Design review of the part built by this model. Coordinates are the model's own, in mm. Face numbers are marked on the shaded views. A direction names the side the tool comes from. Round coordinates to 2 decimals unless told otherwise and drop trailing zeros. Loops run counter-clockwise (first coordinate to the right, second up) from the corner with the lowest first, then second, coordinate; pieces in that order, holes last. Notation, with made-up numbers: (73.5, -13) -> (103.5, -13) arc R18 cw to (103.5, -6) -> close; hole circle Ø7 at (77, 48.25). An arc over 180 degrees is marked (long way). Write each question's results on one line, items separated by ' | '. Start each with the question number.
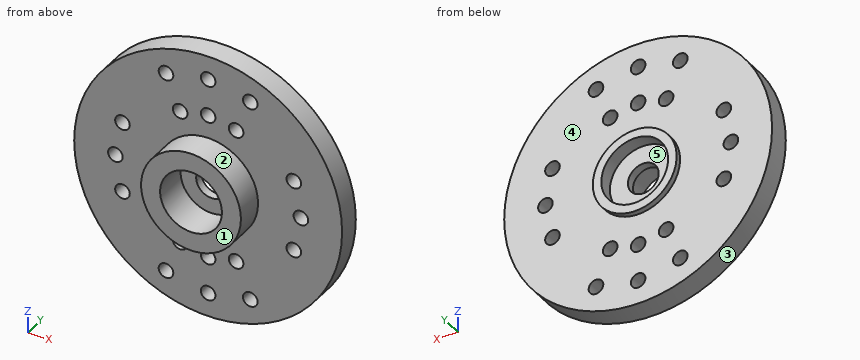
Autodesk Inventor part; units mm, degrees
ref_plane "YZ Plane" through (0, 0, 0) normal (1, 0, 0) x (0, 1, 0)
ref_plane "XZ Plane" through (0, 0, 0) normal (0, 1, 0) x (-1, 0, 0)
ref_plane "XY Plane" through (0, 0, 0) normal (0, 0, 1) x (1, 0, 0)
sketch "Sketch1" plane through (0, 0, 0) normal (0, 1, 0) x (-1, 0, 0)
  circle A0 centre (0, 0) radius 11.915
  dimension "d0" = 23.83
extrude "Extrusion1" add sketch "Sketch1" along normal blind 2
sketch "Sketch2" plane through (0, 2, 0) normal (0, 1, 0) x (1, 0, 0)
  circle A0 centre (0, 6.5) radius 0.65
  line L0 (0, 0) -> (6.5, 0) construction
  circle A1 centre (2.4874, 6.0052) radius 0.65
  circle A2 centre (8.25, 0) radius 0.65
  line L1 (0, 0) -> (8.25, 0) construction
  circle A3 centre (7.622, 3.1571) radius 0.65
  circle A4 centre (0, 9.8) radius 0.65
  line L2 (0, 0) -> (9.8, 0) construction
  circle A5 centre (3.7503, 9.054) radius 0.65
  circle A6 centre (0, 0) radius 11.915
  circle A7 centre (-2.4874, 6.0052) radius 0.65
  circle A8 centre (-8.25, 0) radius 0.65
  circle A9 centre (-7.622, 3.1571) radius 0.65
  circle A10 centre (-3.7503, 9.054) radius 0.65
  circle A11 centre (0, -6.5) radius 0.65
  circle A12 centre (2.4874, -6.0052) radius 0.65
  circle A13 centre (7.622, -3.1571) radius 0.65
  circle A14 centre (0, -9.8) radius 0.65
  circle A15 centre (3.7503, -9.054) radius 0.65
  circle A16 centre (-3.7503, -9.054) radius 0.65
  circle A17 centre (-2.4874, -6.0052) radius 0.65
  circle A18 centre (-7.622, -3.1571) radius 0.65
  dimension "d5" = 1.3
  dimension "d8" = 1.3
  dimension "d10" = 1.3
  dimension "d13" = 1.3
  dimension "d15" = 1.3
  dimension "d18" = 1.3
extrude "Extrusion2" cut sketch "Sketch2" against normal blind 2 contours A0 | A1 | A2 | A3 | A4 | A5 | A7 | A8 | A9 | A10 | A11 | A12 | A13 | A14 | A15 | A16 | A17 | A18
sketch "Sketch3" plane through (0, 2, 0) normal (0, 1, 0) x (1, 0, 0)
  circle A0 centre (0, 0) radius 3.73
  dimension "d21" = 7.46
extrude "Extrusion3" add sketch "Sketch3" along normal blind 0.5
sketch "Sketch4" plane through (0, 2.5, 0) normal (0, 1, 0) x (1, 0, 0)
  circle A0 centre (0, 0) radius 2.97
  dimension "d24" = 5.94
extrude "Extrusion4" cut sketch "Sketch4" against normal blind 1.25
sketch "Sketch5" plane through (0, 1.25, 0) normal (0, 1, 0) x (1, 0, 0)
  circle A0 centre (0, 0) radius 1.37
  dimension "d27" = 2.74
extrude "Extrusion5" cut sketch "Sketch5" against normal blind 0.75
sketch "Sketch6" plane through (0, 0, 0) normal (0, -1, 0) x (1, 0, 0)
  circle A0 centre (0, 0) radius 4.44
  dimension "d30" = 8.88
extrude "Extrusion6" add sketch "Sketch6" along normal blind 2.5
sketch "Sketch7" plane through (0, -2.5, 0) normal (0, -1, 0) x (1, 0, 0)
  circle A0 centre (0, 0) radius 2.75
  dimension "d33" = 5.5
extrude "Extrusion7" cut sketch "Sketch7" against normal blind 3
properties part number "MMAE 232 Assignment 2_White Circle - Dylan Tamras"
1) To check wall thickness, follow line 1 (Z direction, x = 0, y = 1.5) (3 decimals); line 2 (Z direction, x = 0, y = 1.05) (3 decimals); line 3 (Z direction, x = -8, y = 1.25). State the ranges of each line that lie inside material, in increasing order. Write a range as from..to.
2) Take a section at B-B (y = -0.6). Write out the cut boundary in (x, z), plus the area to 3 significant figures.
3) Take a section at C-C (x = 6). Write out the cut boundary in (y, z), plus the area to 3 significant figures.
4) Take a section at A-A (x = 0). State how many separate pieces and enclosed holes the cut face has, plus the area to 3 significant figures.
5) Take a section at D-D (x = -9.75). Write out the cut boundary in (y, z), plus the area to 3 significant figures.
6) The part is to be moulded in two halves that separate along X. For the marked faces 3, 4 and 5, say which applies: +X half, -X half, draft (parallel to the pull), parting line (faces both ways), or undercut.
7) Insertion check: pin 1 (1 mm diameter, centred on x = -2.49, z = -6.01, fed in from -Y); pin 2 (1.5 mm diameter, centred on x = 3.75, z = -9.05, fed in from -Y); pin 3 (1.5 mm diameter, centred on y = 1, z = 7, fed in from -X); pin 4 (4.5 mm diameter, centred on x = -0.5, z = -1, fed in from -Y). Each pin has a flat end and moves straight along its axis. Give the tip position at first contact, or say it passes through.
8) For the marked faces 1 and 2, list the 3-axis set-ups (+Z, -Z, +X, -X, +Y, -Y) from which the entire face can be reached by the end or side of a thin tool; tool diameter is ignored.
Geometry check:
1) line 1: z = -11.915..-10.45, -9.15..-7.15, -5.85..-2.97, 2.97..5.85, 7.15..9.15, 10.45..11.915 | line 2: z = -11.915..-10.45, -9.15..-7.15, -5.85..-1.37, 1.37..5.85, 7.15..9.15, 10.45..11.915 | line 3: z = -8.83..-3.69, -2.63..-0.6, 0.6..2.63, 3.69..8.83
2) outline: circle Ø8.88 at (0, 0); hole circle Ø5.5 at (0, 0) | area: 38.2 mm^2
3) outline: (0, -10.29) -> (2, -10.29) -> (2, 10.29) -> (0, 10.29) -> close | area: 41.2 mm^2
4) separate pieces: 6 | enclosed holes: 0 | area: 37.2 mm^2
5) outline: (0, -6.85) -> (2, -6.85) -> (2, 6.85) -> (0, 6.85) -> close | area: 27.4 mm^2
6) face 3: parting line | face 4: draft | face 5: undercut
7) pin 1: passes through | pin 2: stops at y = 0 | pin 3: stops at x = -10.14 | pin 4: stops at y = -2.5
8) face 1: +Z, -Z, +X, -X, -Y | face 2: -Y
